Print and shaded views of the part. All mm, measured from the part's lowest x, y and z. Coordinates: 2 decimals unless noted, no trailing zeros. Order: outer loops, then holes, each group sorted by start corner. A loop starts at its lowest first (then second) coordinate and runs counter-clockwise, first axis right, second up. Notation, with made-up numbers: (25.5, -36.5) -> (64.5, -36.5) arc R24 cw to (64.5, -19.5) -> close; hole circle Ø7 at (-30.5, -38.75). An arc over 180 degrees is marked (long way). Return JSON: item names as keys, results as strings. Group by question number.
1) Probe line 1 (X direction, y = 4, z = 123); line 2 (Z direction, x = 120, y = 5.5); line 3 (X direction, y = 4.75, z = 54.5). List the from-to ranges inside material, lowest first.
2) Cut at B-B (z = 123). Write the cut outline in (x, y).
3) Cut at D-D (y = 1). State how many separate pieces and enclosed holes the cut face has, and give its area (3 significant figures).
4) Cut at A-A (x = 123). Write the cut outline in (y, z).
5) Flat gauge pin, fed straight in: pin 1 (1 mm diameter, centred on x = 161.5, y = 3.5, fed in from +Z). Where does the tip first touch, or does it go through?
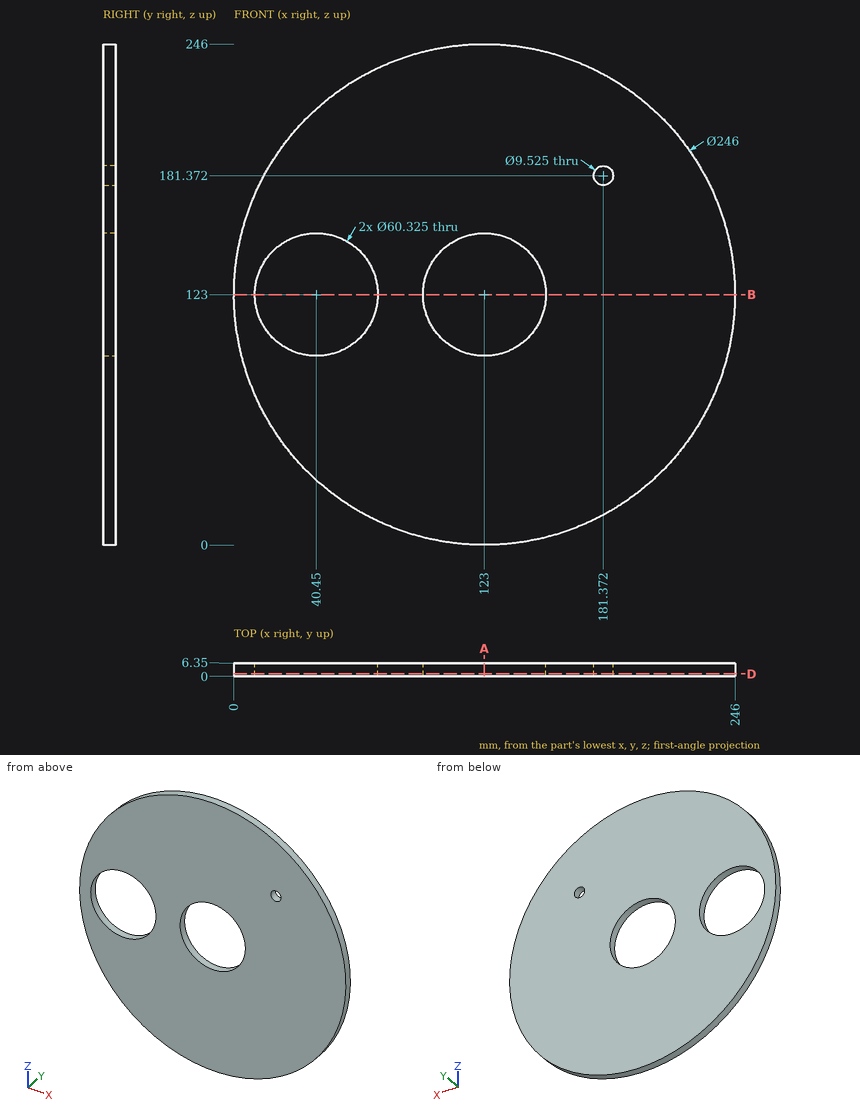
Answers below:
{
 "1": {"line 1": "x = 0 to 10.29, 70.61 to 92.84, 153.16 to 246", "line 2": "z = 0.04 to 92.99, 153.01 to 245.96", "line 3": "x = 20.84 to 225.16"},
 "2": {"outline": "(0, 0) -> (10.29, 0) -> (10.29, 6.35) -> (0, 6.35) -> close; (70.61, 0) -> (92.84, 0) -> (92.84, 6.35) -> (70.61, 6.35) -> close; (153.16, 0) -> (246, 0) -> (246, 6.35) -> (153.16, 6.35) -> close"},
 "3": {"separate pieces": "1", "enclosed holes": "3", "area": "41,700 mm^2"},
 "4": {"outline": "(0, 0) -> (6.35, 0) -> (6.35, 92.84) -> (0, 92.84) -> close; (0, 153.16) -> (6.35, 153.16) -> (6.35, 246) -> (0, 246) -> close"},
 "5": {"pin 1": "stops at z = 239.98"}
}
